```python
from build123d import *

# Parameters (mm, degrees)
SKETCH_1_R          = 1.5
EXTRUDE_1_DEPTH     = 10
EXTRUDE_START       = 1
SKETCH_2_R          = 2.5
SKETCH_2_R_2        = 1.5
EXTRUDE_2_DEPTH     = 1
SKETCH_3_R          = 2.5
SKETCH_3_R_2        = 1.5
EXTRUDE_3_DEPTH     = 1
FILLET_1_R          = 4
SKETCH_6_R          = 1.5
EXTRUDE_4_DEPTH     = 2
SKETCH_7_R          = 1.5
EXTRUDE_5_DEPTH     = 1
EXTRUDE_START_2     = 2
SKETCH_8_R          = 1.5
EXTRUDE_6_DEPTH     = 2
EXTRUDE_7_DEPTH     = 4
SKETCH_10_R         = 4.5
CUT_EXTRUDE_1_DEPTH = 4


with BuildPart() as part:
    # 草图1 → 凸台-拉伸1 (new body)
    with BuildSketch(Plane.XY):
        with BuildLine():
            Line((4, 0), (13, 0))
            ThreePointArc((13, 0), (15.5, 2.5), (13, 5))
            Line((13, 5), (4, 5))
            Line((4, 5), (4, 24.5))
            Line((4, 24.5), (16, 24.5))
            Line((16, 24.5), (16, 26.5))
            Line((16, 26.5), (0, 26.5))
            Line((0, 26.5), (0, 4))
            ThreePointArc((0, 4), (1.171572875, 1.171572875), (4, 0))
        make_face()
        with Locations((13, 2.5)):
            Circle(SKETCH_1_R, mode=Mode.SUBTRACT)
    extrude(amount=EXTRUDE_1_DEPTH)

    # 草图2 → 凸台-拉伸2 (add)
    with BuildSketch(Plane(origin=(0, 0, 0), x_dir=(-1, 0, 0), z_dir=(0, 0, -1)).offset(EXTRUDE_START)):
        with Locations((-13, 2.5)):
            Circle(SKETCH_2_R)
        with Locations((-13, 2.5)):
            Circle(SKETCH_2_R_2, mode=Mode.SUBTRACT)
    extrude(amount=-EXTRUDE_2_DEPTH)

    # 草图3 → 凸台-拉伸3 (add)
    with BuildSketch(Plane.XY.offset(10)):
        with Locations(Location((13, 2.5, 0), (0, 0, 180))):
            Circle(SKETCH_3_R)
        with Locations(Location((13, 2.5, 0), (0, 0, 180))):
            Circle(SKETCH_3_R_2, mode=Mode.SUBTRACT)
    extrude(amount=EXTRUDE_3_DEPTH)

    # 圆角1
    fillet_1_edges = [part.edges().sort_by_distance(p)[0] for p in [
        (16, 25.5, 10),
        (16, 25.5, 0),
    ]]
    fillet(fillet_1_edges, radius=FILLET_1_R)

    # 草图6 → 凸台-拉伸4 (add)
    with BuildSketch(Plane.XZ.offset(-24.5)):
        with Locations(Location((12.5, 5, 0), (0, 0, 180))):
            Circle(SKETCH_6_R)
    extrude(amount=EXTRUDE_4_DEPTH)

    # 草图7 → 凸台-拉伸5 (add, symmetric)
    with BuildSketch(Plane(origin=(0, 5, 0), x_dir=(1, 0, 0), z_dir=(0, 1, 0))):
        with Locations(Location((12.5, -5, 0), (0, 0, 180))):
            Circle(SKETCH_7_R)
    extrude(amount=EXTRUDE_5_DEPTH, both=True)

    # 草图8 → 凸台-拉伸6 (add)
    with BuildSketch(Plane(origin=(0, 6, 0), x_dir=(1, 0, 0), z_dir=(0, 1, 0)).offset(EXTRUDE_START_2)):
        with Locations(Location((12.5, -5, 0), (0, 0, 180))):
            Circle(SKETCH_8_R)
    extrude(amount=-EXTRUDE_6_DEPTH)

    # 草图9 → 凸台-拉伸7 (add)
    with BuildSketch(Plane.ZY):
        with BuildLine():
            Line((10, 26.5), (11.923076923, 18.884615385))
            ThreePointArc((11.923076923, 18.884615385), (12.5, 16), (11.923076923, 13.115384615))
            Line((11.923076923, 13.115384615), (10, 4))
            Line((10, 4), (0, 4))
            Line((0, 4), (-1.923076923, 13.115384615))
            ThreePointArc((-1.923076923, 13.115384615), (-2.5, 16), (-1.923076923, 18.884615385))
            Line((-1.923076923, 18.884615385), (0, 26.5))
            Line((0, 26.5), (10, 26.5))
        make_face()
    extrude(amount=-EXTRUDE_7_DEPTH)

    # 草图10 → 切除-拉伸1 (cut)
    with BuildSketch(Plane.ZY):
        with Locations(Location((5, 16, 0), (0, 0, 270))):
            Circle(SKETCH_10_R)
    extrude(amount=-CUT_EXTRUDE_1_DEPTH, mode=Mode.SUBTRACT)

    # 草图11 → 旋转1 (revolve)
    with BuildSketch(Plane.ZY.offset(-12.5), mode=Mode.PRIVATE) as revolve_1_sk:
        with BuildLine():
            Line((5, 26.5), (3, 26.5))
            Line((3, 26.5), (3.913470068, 27.641837585))
            ThreePointArc((3.913470068, 27.641837585), (3.358750534, 29.575719227), (5, 30.739296536))
            Line((5, 30.739296536), (5, 29))
            Line((5, 29), (5, 26.5))
        make_face()
    revolve(revolve_1_sk.sketch.rotate(Axis((12.5, 29, 5), (0, 1, 0)), 340.52877936), axis=Axis((12.5, 29, 5), (0, 1, 0)))


solid = part.part
```
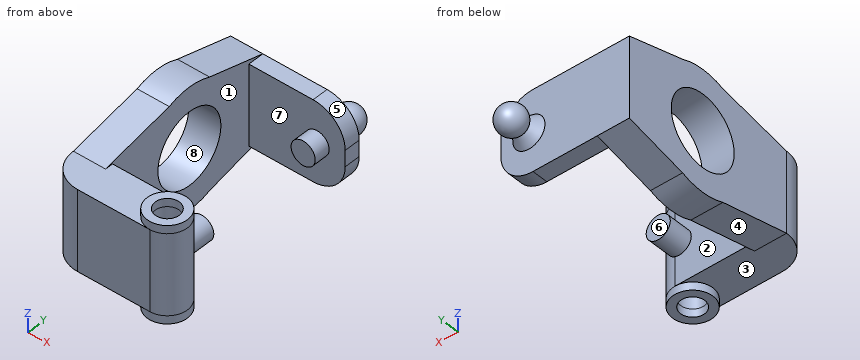
Geometry: final body of the model. Coordinates: model frame, mm. Face numbers are marked on the shaded views. A direction names the side the tool comes from. Coordinates: 2 decimals unless noted, no trailing zeros. Order: outer loops, then holes, each group sorted by start corner. A loop starts at its lowest first (then second) coordinate and runs counter-clockwise, first axis right, second up. Notation, with made-up numbers: (32.5, 79) -> (85.5, 79) arc R31 ccw to (85.5, 116) -> close; hole circle Ø3 at (29.5, 16.25). An arc over 180 degrees is marked (long way). Write each question's results on one line, items separated by ' | '. Start each with the question number.
1) Cut plane D-D, the plane x = 12.5. State how many separate pieces and enclosed holes the cut face has, and give its area (3 significant figures).
2) Cut plane C-C, the plane z = 8.75. Output: boundary loops of the cut face in (x, y).
3) Mould query, pull axis Y, two halves, no side actions, for the marked faces 1, 2, 3 and 4. Classes: released by +Y, released by -Y, zero draft, split by the parting line, or undercut.
4) Material intervals for line 1 along Y through (x, z) = (13, 7.5); line 2 along Y through (x, z) = (13, 10.4); line 3 along Y through (x, z) = (12.25, 1.25), sorted ascending.
5) First-contact query: pin 1 (4 mm diameter, centred on x = 9.5, y = 2.5, fed in from +Z); pin 2 (5 mm diameter, centred on x = 13, y = 2.5, fed in from -Z); pin 3 (2 mm diameter, centred on x = 8, y = 26, fed in from -Z). Flat tips, straight axial feed; report the tip coordinate or a pass-through.
6) Cut plane B-B, the plane x = 4.5. Output: boundary loops of the cut face in (y, z).
7) Cut plane A-A, the plane y = 16. Output: boundary loops of the cut face in (x, z), and give its area (3 significant figures).
8) Set-up query: the marked faces 5, 6, 7 and 8. Return all of +Z, -Z, +X, -X, +Y, -Y with unobstructed straight access to the full face (end or side cutting, diameter ignored); none if empty.
Checks:
1) separate pieces: 3 | enclosed holes: 0 | area: 73.2 mm^2
2) outline: (0, 4) arc R4 ccw to (4, 0) -> (13, 0) arc R2.5 ccw to (13, 5) -> (4, 5) -> (4, 13.51) -> (0, 13.51) -> close; (0, 18.49) -> (4, 18.49) -> (4, 24.5) -> (14.9, 24.5) -> (14.9, 26.5) -> (0, 26.5) -> close; hole circle Ø3 at (13, 2.5)
3) face 1: undercut | face 2: undercut | face 3: zero draft | face 4: released by -Y
4) line 1: 0 to 1, 4 to 5, 24.5 to 26.5 | line 2: 0 to 1, 4 to 5 | line 3: 0 to 1.2, 3.8 to 5, 24.5 to 26.5
5) pin 1: z = 11 | pin 2: z = -1 | pin 3: z = 0
6) outline: (0, 0) -> (5, 0) -> (5, 10) -> (0, 10) -> close; (24.5, 0) -> (26.5, 0) -> (26.5, 10) -> (24.5, 10) -> close
7) outline: (0, -2.5) -> (4, -2.5) -> (4, 0.5) -> (0, 0.5) -> close; (0, 9.5) -> (4, 9.5) -> (4, 12.5) -> (0, 12.5) -> close | area: 24.0 mm^2
8) face 5: +Z, +X, +Y | face 6: +Z, -Z, +X | face 7: none | face 8: +X, -X
